Here's how the part is built. I have some questions about the finished solid (model axes, mm). A direction names the side the tool comes from. Round coordinates to 2 decimals unless told otherwise and drop trailing zeros. Write each loop counter-clockwise with the first axis right and the second up, starting at its lowest first coordinate (ties: lowest second). Pieces come first, ordered by that corner, then holes. Notation, with made-up numbers: M 26.5,53.5 L 70.5,53.5 A10 ccw 70.5,61.5 Z; hole C 2.25,8 d3. An arc over 180 degrees is marked long. Use one line per item in the form item = value. Start each with the question number.
Q1. I want a section at D-D on x = 152.5. List the corners of the cut face in (y, z) for me, and give its area (3 significant figures).
Q2. I want a section at A-A on z = 33. List the corners of the cut face in (x, y) for me.
Q3. I want a section at C-C on y = 30. List the corners of the cut face in (x, z) for me, and give its area (3 significant figures).
Q4. We'd pull the mould along X, two halves only. Please class faces 1 (the face through (103, 17, 62.738)), 2 (the face through (157.95, 62.93, 28.93)), 3 (the face through (87.921, 42, 82)), 4 (the face through (100, 0, 31)): +X half, -X half, draft (parallel to the pull), parting line (faces both ways), or undercut.
Q5. I need wall thicknesses on line 1 along X through (y, z) = (31.5, 93.5); line 2 along X through (y, z) = (65, 85.5); line 3 along Z through (x, y) = (20, 9). Which ranges of each line are inside material? Lowest first, please. Write a range as from..to.
Q6. I want a section at B-B on x = 22. List the corners of the cut face in (y, z) for me.
Q7. For faces 5 (the face through (37.121, 42, 82)), 6 (the face through (19, 20.574, 82)), 7 (the face through (37.084, 78, 58)), which set-ups out of +Z, -Z, +X, -X, +Y, -Y let a thin tool reach every point of the face, with its end or its side?
Q8. I'm going to push flat-ended pins straight in: pin 1 Ø6 at (x, z) = (154, 35) entering from +Y; pin 2 Ø10 at (x, z) = (160, 19) entering from +Y; pin 3 Ø18.5 at (x, z) = (20.5, 85) entering from -Y. Where does each tip first touch, or does it pass through?
Autodesk Inventor part; units mm, degrees
ref_plane "YZ Plane" through (0, 0, 0) normal (1, 0, 0) x (0, 1, 0)
ref_plane "XZ Plane" through (0, 0, 0) normal (0, 1, 0) x (-1, 0, 0)
ref_plane "XY Plane" through (0, 0, 0) normal (0, 0, 1) x (1, 0, 0)
sketch "Sketch1" plane through (0, 0, 0) normal (0, 0, 1) x (1, 0, 0)
  line L0 (0, 0) -> (203.2, 0)
  line L1 (203.2, 0) -> (203.2, 101.6)
  line L2 (203.2, 101.6) -> (0, 101.6)
  line L3 (0, 101.6) -> (0, 0)
  dimension "d0" = 203.2
  dimension "d1" = 101.6
extrude "Extrusion1" add sketch "Sketch1" along normal blind 101.6
sketch "Sketch2" plane through (203.2, 0, 0) normal (1, 0, 0) x (0, 0, -1)
  line L0 (0, 0) -> (-101.6, 0)
  line L1 (-101.6, 0) -> (-62.738, 0)
  line L2 (-62.738, 0) -> (-101.6, 0)
  line L3 (-62.738, 0) -> (-62.738, 20.574)
  line L4 (-62.738, 20.574) -> (-101.6, 20.574)
  line L5 (-101.6, 0) -> (-101.6, 101.6)
  line L6 (-101.6, 20.574) -> (-101.6, 0)
  dimension "d4" = 38.862
  dimension "d5" = 20.574
extrude "Extrusion2" cut sketch "Sketch2" against normal blind 203.2
sketch "Sketch3" plane through (0, 101.6, 0) normal (0, 1, 0) x (1, 0, 0)
  line L0 (0, 0) -> (0, -101.6)
  line L1 (0, -101.6) -> (37.084, -101.6)
  line L2 (203.2, -101.6) -> (0, -101.6)
  line L3 (37.084, -101.6) -> (37.084, -29.464)
  line L4 (37.084, -29.464) -> (159.766, -29.464)
  line L5 (159.766, -29.464) -> (159.766, -101.6)
  dimension "d8" = 37.084
  dimension "d9" = 72.136
  dimension "d10" = 122.682
sketch "Sketch4" plane through (0, 101.6, 0) normal (0, 1, 0) x (1, 0, 0)
  line L0 (203.2, -101.6) -> (0, -101.6)
  line L1 (37.1206, -101.6) -> (-1.7414, -101.6)
  line L2 (37.1206, -101.6) -> (37.1206, -62.738)
  line L3 (37.1206, -62.738) -> (87.9206, -62.738)
  line L4 (203.2, -62.738) -> (0, -62.738)
  line L5 (87.9206, -62.738) -> (87.9206, -101.6)
  point P0 (0, 0)
  dimension "d11" = 38.862
  dimension "d12" = 38.862
  dimension "d13" = 50.8
extrude "Extrusion3" cut sketch "Sketch4" against normal blind 203.2
extrude "Extrusion4" cut sketch "Sketch3" against normal blind 39.624
sketch "Sketch5" plane through (0, 0, 101.6) normal (0, 0, 1) x (1, 0, 0)
  line L0 (203.2, 20.574) -> (203.2, 101.6)
  line L1 (203.2, 101.6) -> (203.2, 37.592)
  line L2 (203.2, 37.592) -> (203.2, 101.6)
  line L3 (203.2, 101.6) -> (88.9, 101.6)
  line L4 (203.2, 101.6) -> (0, 101.6)
  line L5 (88.9, 101.6) -> (203.2, 37.592)
  point P0 (0, 0)
  dimension "d18" = 64.008
  dimension "d19" = 114.3
extrude "Extrusion5" cut sketch "Sketch5" against normal blind 101.6
sketch "Sketch6" plane through (0, 0, 101.6) normal (0, 0, 1) x (1, 0, 0)
  point P0 (0, 0)
sketch "Sketch7" plane through (0, 101.6, 101.6) normal (0, 1, 0) x (1, 0, 0)
  line L0 (37.084, 0) -> (0, 0)
  line L1 (0, 0) -> (0, 38.862)
  line L2 (0, 101.6) -> (0, 0)
  dimension "d22" = 38.862
sketch "Sketch8" plane through (0, 0, 0) normal (-1, 0, 0) x (0, 0, 1)
  point P0 (0, 0)
sketch "Sketch9" plane through (0, 0, 0) normal (-1, 0, 0) x (0, 0, 1)
  line L0 (101.6, 101.6) -> (101.6, 20.574)
  line L1 (101.6, 101.6) -> (101.6, 61.976)
  line L2 (101.6, 61.976) -> (62.8835, 101.6)
  line L3 (101.6, 101.6) -> (29.464, 101.6)
  line L4 (62.8835, 101.6) -> (101.6, 101.6)
  point P0 (0, 0)
  dimension "d23" = 39.624
extrude "Extrusion6" cut sketch "Sketch9" against normal blind 101.6
properties part number "orthographic4"
Reported:
q1.outline = M 0,0 L 65.98,0 L 65.98,29.46 L 61.98,29.46 L 61.98,101.6 L 20.57,101.6 L 20.57,62.74 L 0,62.74 Z
q1.area = 5,620 mm^2
q2.outline = M 0,0 L 203.2,0 L 203.2,37.59 L 159.66,61.98 L 37.08,61.98 L 37.08,101.6 L 0,101.6 Z
q3.outline = M 0,0 L 203.2,0 L 203.2,101.6 L 87.92,101.6 L 87.92,62.74 L 37.12,62.74 L 37.12,101.6 L 0,101.6 Z
q3.area = 18,700 mm^2
q4.face_1 = undercut
q4.face_2 = +X half
q4.face_3 = undercut
q4.face_4 = draft
q5.line_1 = 0..37.12, 87.92..203.2
q5.line_2 = 0..37.08
q5.line_3 = 0..62.74
q6.outline = M 0,0 L 101.6,0 L 101.6,62.88 L 61.98,101.6 L 20.57,101.6 L 20.57,62.74 L 0,62.74 Z
q7.face_5 = +Z, +Y, -Y
q7.face_6 = +Z, +X, -X, -Y
q7.face_7 = +Z, +X, +Y
q8.pin_1 = 61.98
q8.pin_2 = 64.58
q8.pin_3 = 20.57
